Here's how the part is built. I have some questions about the finished solid (model axes, mm). A direction names the side the tool comes from. Coordinates: 2 decimals unless noted, no trailing zeros. Order: outer loops, then holes, each group sorted by start corner. A loop starts at its lowest first (then second) coordinate and runs counter-clockwise, first axis right, second up. Notation, with made-up numbers: (20.25, -20) - (58.25, -20) arc R19 cw to (58.25, 4) - close; hole circle Ø1 at (-22, 61). An arc over 180 degrees is marked (long way). Use one line per item in the form item = value. Start each with the question number.
from build123d import *

# Parameters (mm, degrees)
SKETCH1_W                      = 300
SKETCH1_H                      = 1300
BASE_FLANGE1_DEPTH             = 10
EDGE_FLANGE1_STRIP_W           = 68
EDGE_FLANGE1_STRIP_H           = 10
EDGE_FLANGE1_STRIP_CUT_DEPTH   = 1300
EDGE_FLANGE1_STRIP_2_W         = 68
EDGE_FLANGE1_STRIP_2_H         = 10
EDGE_FLANGE1_STRIP_CUT_2_DEPTH = 1300
EDGE_FLANGE1_DEPTH             = 1300
EDGE_FLANGE1_BEND_DEPTH        = 1300
SKETCH12_R                     = 9.5
CUT_EXTRUDE1_DEPTH             = 10
MIRROR2_COPY_1_SKETCH_R        = 9.5
MIRROR2_COPY_1_DEPTH           = 10
SKETCH13_R                     = 27.5
CUT_EXTRUDE2_DEPTH             = 10
LPATTERN1_COUNT                = 3
LPATTERN1_PITCH                = 310
SKETCH14_R                     = 10
CUT_EXTRUDE3_DEPTH             = 732.436941916
LPATTERN2_COUNT                = 7
LPATTERN2_PITCH                = 152
SKETCH18_R                     = 10
CUT_EXTRUDE4_DEPTH             = 732.436941916
SKETCH20_R                     = 9
CUT_EXTRUDE5_DEPTH             = 10


# Sheet-metal steps are written as plain solids
with BuildPart() as part:
    # Sketch1 → Base-Flange1 (new body)
    with BuildSketch(Plane(origin=(0, 0, 0), x_dir=(0, 0, -1), z_dir=(1, 0, 0))):
        Rectangle(SKETCH1_W, SKETCH1_H)
    extrude(amount=-BASE_FLANGE1_DEPTH)

    # Edge-Flange1 strip (across the edge) → Edge-Flange1 strip cut (cut)
    with BuildSketch(Plane(origin=(-10, -650, 150), x_dir=(0, 0, -1), z_dir=(0, 1, 0))):
        with Locations((-10, -5)):
            Rectangle(EDGE_FLANGE1_STRIP_W, EDGE_FLANGE1_STRIP_H)
    extrude(amount=EDGE_FLANGE1_STRIP_CUT_DEPTH, mode=Mode.SUBTRACT)

    # Edge-Flange1 strip 2 (across the edge) → Edge-Flange1 strip cut 2 (cut)
    with BuildSketch(Plane(origin=(-10, 650, -150), x_dir=(0, 0, 1), z_dir=(0, -1, 0))):
        with Locations((-10, -5)):
            Rectangle(EDGE_FLANGE1_STRIP_2_W, EDGE_FLANGE1_STRIP_2_H)
    extrude(amount=EDGE_FLANGE1_STRIP_CUT_2_DEPTH, mode=Mode.SUBTRACT)

    # Edge-Flange1 section (across the edge) → Edge-Flange1 (add)
    with BuildSketch(Plane(origin=(-10, -650, 150), x_dir=(0, 0, -1), z_dir=(0, 1, 0))):
        with BuildLine():
            Line((0, 14), (0, 140))
            Line((0, 140), (10, 140))
            Line((10, 140), (10, 14))
            ThreePointArc((10, 14), (14.100505063, 4.100505063), (24, 0))
            Line((24, 0), (24, -10))
            ThreePointArc((24, -10), (7.029437252, -2.970562748), (0, 14))
        make_face()
    extrude(amount=EDGE_FLANGE1_DEPTH)

    # Edge-Flange1 section 2 (across the edge) → Edge-Flange1 bend (add)
    with BuildSketch(Plane(origin=(-10, 650, -150), x_dir=(0, 0, 1), z_dir=(0, -1, 0))):
        with BuildLine():
            Line((0, 14), (0, 140))
            Line((0, 140), (10, 140))
            Line((10, 140), (10, 14))
            ThreePointArc((10, 14), (14.100505063, 4.100505063), (24, 0))
            Line((24, 0), (24, -10))
            ThreePointArc((24, -10), (7.029437252, -2.970562748), (0, 14))
        make_face()
    extrude(amount=EDGE_FLANGE1_BEND_DEPTH)

    # Sketch12 → Cut-Extrude1 (cut)
    with BuildSketch(Plane(origin=(0, 0, 0), x_dir=(0, 0, -1), z_dir=(1, 0, 0))):
        with Locations((90, 580)):
            Circle(SKETCH12_R)
        with Locations((0, 580)):
            Circle(SKETCH12_R)
    cut_extrude1 = extrude(amount=-CUT_EXTRUDE1_DEPTH, mode=Mode.SUBTRACT)

    # Mirror1: Cut-Extrude1 across plane
    add(cut_extrude1.mirror(Plane.ZX), mode=Mode.SUBTRACT)

    # Mirror2: Cut-Extrude1 across plane
    add(cut_extrude1.mirror(Plane.XY), mode=Mode.SUBTRACT)

    # Mirror2 copy 1 sketch → Mirror2 copy 1 (cut)
    with BuildSketch(Plane(origin=(0, 0, 0), x_dir=(0, 0, 1), z_dir=(1, 0, 0))):
        with Locations((90, 580)):
            Circle(MIRROR2_COPY_1_SKETCH_R)
        with Locations((0, 580)):
            Circle(MIRROR2_COPY_1_SKETCH_R)
    extrude(amount=-MIRROR2_COPY_1_DEPTH, mode=Mode.SUBTRACT)

    # Sketch13 → Cut-Extrude2 (cut)
    with BuildSketch(Plane(origin=(0, 0, 0), x_dir=(0, 0, -1), z_dir=(1, 0, 0))):
        with Locations((0, 310)):
            Circle(SKETCH13_R)
    cut_extrude2 = extrude(amount=-CUT_EXTRUDE2_DEPTH, mode=Mode.SUBTRACT)

    # LPattern1: Cut-Extrude2 ×3
    with Locations(*[(0, -i * LPATTERN1_PITCH, 0) for i in range(1, LPATTERN1_COUNT)]):
        add(cut_extrude2, mode=Mode.SUBTRACT)

    # Sketch14 → Cut-Extrude3 (cut, through all)
    with BuildSketch(Plane(origin=(0, 0, -150), x_dir=(-1, 0, 0), z_dir=(0, 0, -1))):
        with Locations((87, -456)):
            Circle(SKETCH14_R)
    cut_extrude3 = extrude(amount=-CUT_EXTRUDE3_DEPTH, mode=Mode.SUBTRACT)

    # LPattern2: Cut-Extrude3 ×7
    with Locations(*[(0, i * LPATTERN2_PITCH, 0) for i in range(1, LPATTERN2_COUNT)]):
        add(cut_extrude3, mode=Mode.SUBTRACT)

    # Sketch18 → Cut-Extrude4 (cut, through all)
    with BuildSketch(Plane(origin=(0, 0, -150), x_dir=(-1, 0, 0), z_dir=(0, 0, -1))):
        with Locations((45, 545)):
            Circle(SKETCH18_R)
        with Locations((45, 585)):
            Circle(SKETCH18_R)
        with Locations((45, 30)):
            Circle(SKETCH18_R)
    cut_extrude4 = extrude(amount=-CUT_EXTRUDE4_DEPTH, mode=Mode.SUBTRACT)

    # Mirror3: Cut-Extrude4 across plane
    add(cut_extrude4.mirror(Plane.ZX), mode=Mode.SUBTRACT)

    # Sketch20 → Cut-Extrude5 (cut)
    with BuildSketch(Plane(origin=(0, 0, 0), x_dir=(0, 0, -1), z_dir=(1, 0, 0))):
        with Locations((104.55, -370)):
            Circle(SKETCH20_R)
        with Locations((104.55, -460)):
            Circle(SKETCH20_R)
    extrude(amount=-CUT_EXTRUDE5_DEPTH, mode=Mode.SUBTRACT)


solid = part.part
1) I need wall thicknesses on probe 1 along Y at (x, z) = (-6, -90); probe 2 along Z at (x, y) = (-114, -500); probe 3 along Y at (x, z) = (-3, 0). Which ranges of each line are inside material? Lowest first, please. Write a range as [from, to].
2) For pin 1 (2 mm diameter, centred on x = -17.5, y = 111, fed in from +Z); pin 2 (18 mm diameter, centred on x = -45, y = -545, fed in from +Z); pin 3 (23.5 mm diameter, centred on y = -460, z = -104.55, fed in from -X), each with a flat end and sliding along its axis, tell me the tip position at first contact or that it passes through.
3) Suppose I cut it at B-B, the plane y = 403. List the corners of the cut face in (x, z) for me.
4) If we mould it in two halves opening along Z, with no side actions, what happens to faces 3 (the flat face through (0, 9.1, -26.2)), 4 (the flat face through (-102, -9, 140)), 5 (the flat face through (-100, 9, -150))? For each: pulls with the +Z half, pulls with the -Z half, needs draft (parallel to the pull), parting line crosses it, or undercut.
5) Suppose I cut it at A-A, the plane x = -114.5. List the corners of the cut face in (y, z) for me.
6) Which directions (+Z, -Z, +X, -X, +Y, -Y) give clear straight access to the entire face, cutting with the end or side of a thin tool? Please do faces 1 (the flat face through (-9, 650, 1)), 2 (the flat face through (-102, 9, -140)).
From the geometry:
q1.probe_1 = [-650, -589.5], [-570.5, 570.5], [589.5, 650]
q1.probe_2 = [-150, -140], [140, 150]
q1.probe_3 = [-650, -589.5], [-570.5, -337.5], [-282.5, -27.5], [27.5, 282.5], [337.5, 570.5], [589.5, 650]
q2.pin_1 = 149.36
q2.pin_2 = through
q2.pin_3 = -10
q3.outline = (-150, -150) - (-24, -150) arc R24 ccw to (0, -126) - (0, 126) arc R24 ccw to (-24, 150) - (-150, 150) - (-150, 140) - (-24, 140) arc R14 cw to (-10, 126) - (-10, -126) arc R14 cw to (-24, -140) - (-150, -140) - close
q4.face_3 = needs draft
q4.face_4 = undercut
q4.face_5 = pulls with the -Z half
q5.outline = (-650, -150) - (650, -150) - (650, -140) - (-650, -140) - close; (-650, 140) - (650, 140) - (650, 150) - (-650, 150) - close
q6.face_1 = +Z, -Z, +X, -X, +Y
q6.face_2 = -X, +Y, -Y
